The figure shows three views and two pictorial views of one solid part (mm, origin at its lowest corner). Answer the questions. Coordinates: 2 decimals unless noted, no trailing zeros. Order: outer loops, then holes, each group sorted by start corner. A loop starts at its lowest first (then second) coordinate and runs counter-clockwise, first axis right, second up. Notation, with made-up numbers: M 52,38.5 L 91,38.5 A22 ccw 91,51.5 Z; hole C -39,76.25 d11. An arc over 180 degrees is marked long. Use a Markdown table: item, result.
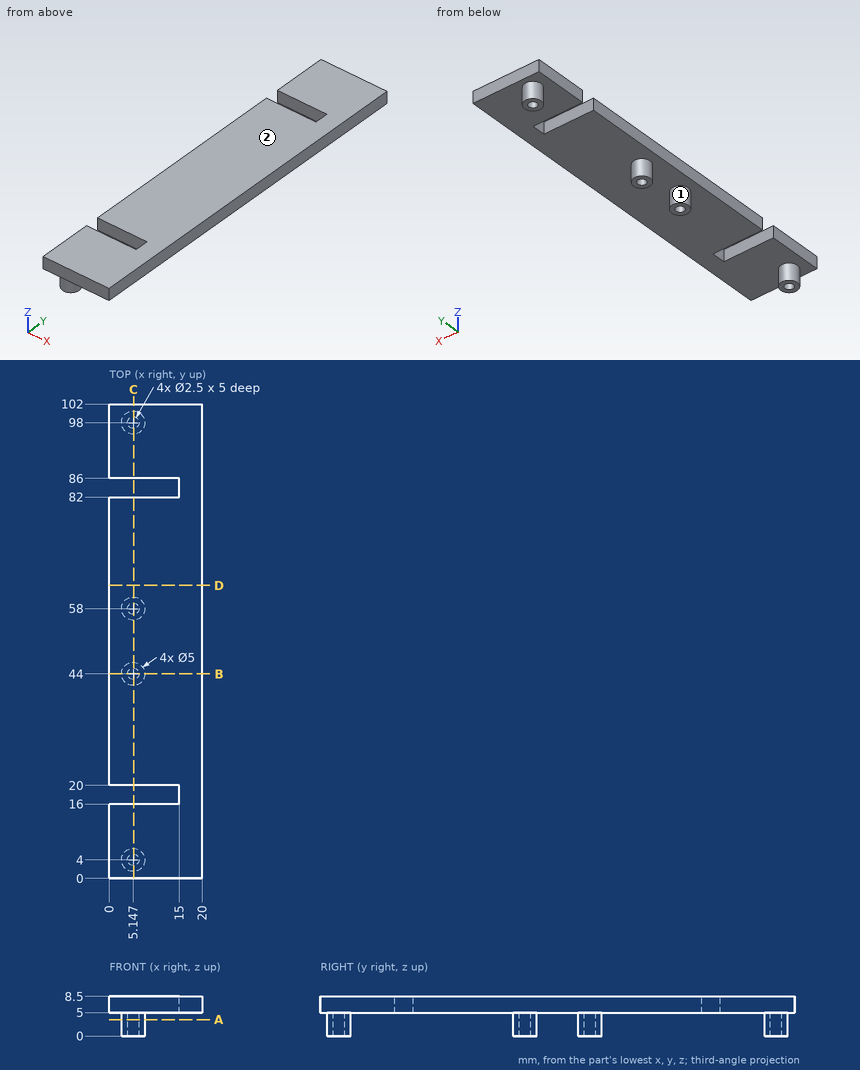
1. Section D-D on y = 63 is taken. Determine the outline of the cut face in (x, z), then the cut area to 3 significant figures.
Answers below:
| item | result |
|---|---|
| outline | M 0,5 L 20,5 L 20,8.5 L 0,8.5 Z |
| area | 70.0 mm² |
2. Flat-ended cylindrical pins translate along their axes: P1, Ø2, axis at x = 16.5, y = 16.5, coming from the -Z side; P2, Ø1, axis at y = 83.5, z = 6.5, coming from the -X side. Find the tip coordinate at first contact, or state that the pin passes through.
Answers below:
| item | result |
|---|---|
| P1 | z = 5 |
| P2 | x = 15 |
3. Section A-A on z = 3.5 is taken. Determine the outline of the cut face in (x, y).
Answers below:
| item | result |
|---|---|
| outline | C 5.15,4 d5; C 5.15,44 d5; C 5.15,58 d5; C 5.15,98 d5; hole C 5.15,4 d2.5; hole C 5.15,44 d2.5; hole C 5.15,58 d2.5; hole C 5.15,98 d2.5 |
4. For a pull along Y with two mould halves and no side action, classify the marked faces 1 and 2 as +Y half, -Y half, draft (parallel to the pull), parting line (faces both ways), or undercut.
Answers below:
| item | result |
|---|---|
| face 1 | undercut |
| face 2 | draft |
5. Find the intervals of material crossed by probe 1 along Y at (x, z) = (2.25, 8); probe 2 along X at (y, z) = (98, 3.5); probe 3 along Z at (x, y) = (8.25, 26.5), in increasing order.
Answers below:
| item | result |
|---|---|
| probe 1 | 0 to 16, 20 to 82, 86 to 102 |
| probe 2 | 2.65 to 3.9, 6.4 to 7.65 |
| probe 3 | 5 to 8.5 |
6. Section C-C on x = 5.25 is taken. Give the number of separate pieces and of enclosed holes in the cut face, then the cut area to 3 significant figures.
Answers below:
| item | result |
|---|---|
| separate pieces | 3 |
| enclosed holes | 0 |
| area | 379 mm² |
7. Section B-B on y = 44 is taken. Determine the outline of the cut face in (x, z).
Answers below:
| item | result |
|---|---|
| outline | M 0,5 L 2.65,5 L 2.65,0 L 3.9,0 L 3.9,5 L 6.4,5 L 6.4,0 L 7.65,0 L 7.65,5 L 20,5 L 20,8.5 L 0,8.5 Z |
